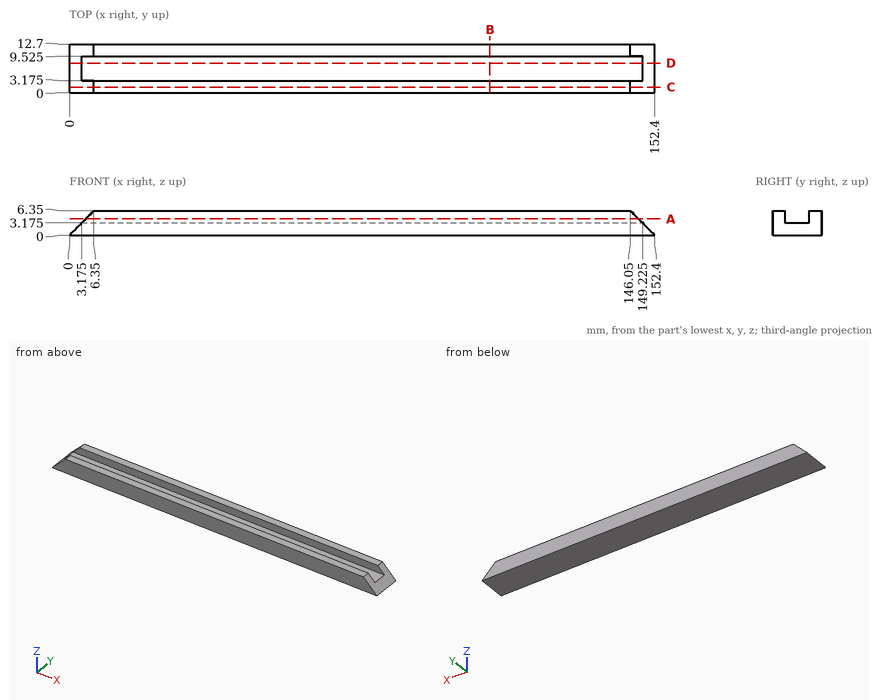
Check sheet for the drawn part. Datum: minimum x, y, z corner. Units: mm. Give positions to 0.01 mm unless a question says otherwise; leave off trailing zeros. Write each loop counter-clockwise with the first axis right and the second up, starting at its lowest first coordinate (ties: lowest second). Pieces come first, ordered by that corner, then holes.
(1) Cross-section at A-A (z = 4.25). Enter the section's corners in (x, y) (3 decimals).
(2) Material ranges on line 1 (Y direction, x = 12.5, z = 5.25) (3 decimals); line 2 (Z direction, x = 142.5, y = 6.75) (3 decimals); line 3 (X direction, y = 11, z = 5), recorded low to high.
(3) Cross-section at B-B (x = 109.5). Enter the section's corners in (y, z) (3 decimals), plus the area to 3 significant figures.
(4) Gauge pin test, flat ends, axial feed: pin 1 (1.9 mm diameter, centred on x = 58.5, y = 6.5, fed in from +Z) (3 decimals); pin 2 (1.5 mm diameter, centred on y = 5.5, z = 3, fed in from -X). Record the tip position at first contact, or that the pin passes through.
(5) Cross-section at C-C (y = 1.5). Enter the section's corners in (x, z).
(6) Cross-section at D-D (y = 7.75). Enter the section's corners in (x, z) (3 decimals), plus the area to 3 significant figures.
Worked out:
1. outline: (4.25, 0) - (148.15, 0) - (148.15, 3.175) - (4.25, 3.175) - close; (4.25, 9.525) - (148.15, 9.525) - (148.15, 12.7) - (4.25, 12.7) - close
2. line 1: y = 0 to 3.175, 9.525 to 12.7
2. line 2: z = 0 to 3.175
2. line 3: x = 5 to 147.4
3. outline: (0, 0) - (12.7, 0) - (12.7, 6.35) - (9.525, 6.35) - (9.525, 3.175) - (3.175, 3.175) - (3.175, 6.35) - (0, 6.35) - close
3. area: 60.5 mm2
4. pin 1: stops at z = 3.175
4. pin 2: stops at x = 2.25
5. outline: (0, 0) - (152.4, 0) - (146.05, 6.35) - (6.35, 6.35) - close
6. outline: (0, 0) - (152.4, 0) - (149.225, 3.175) - (3.175, 3.175) - close
6. area: 474 mm2
